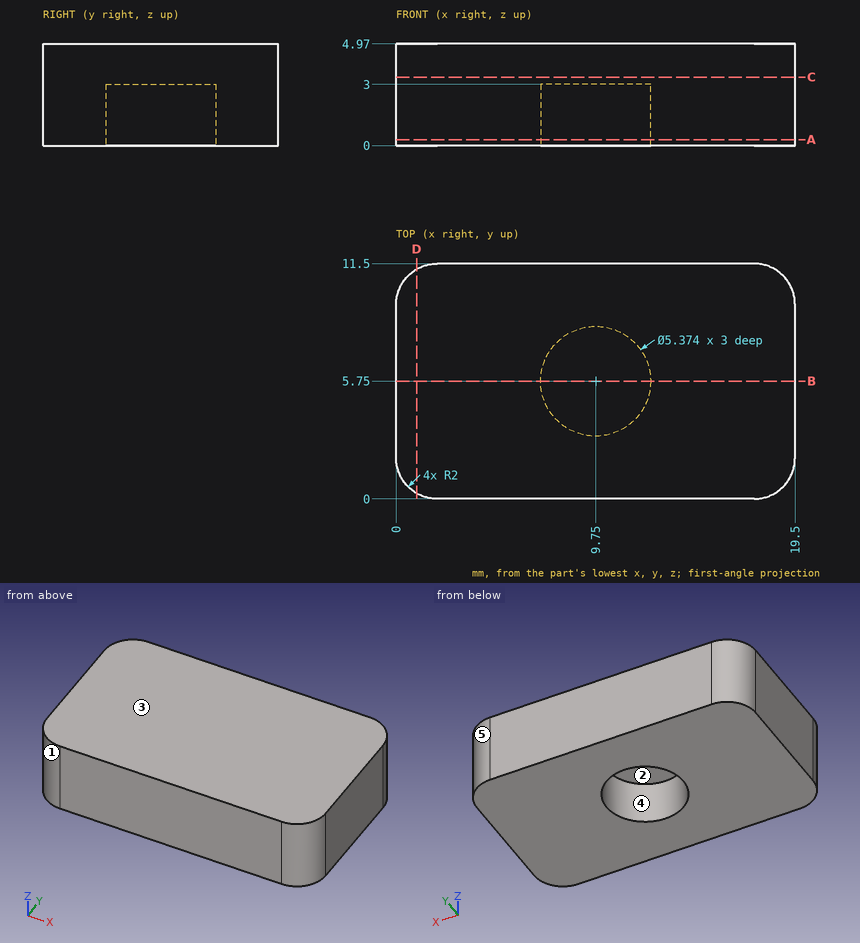
Job drawing, mm, ordinate dimensions from the low corner. One solid piece. A direction names the side the tool comes from. Coordinates: 2 decimals unless noted, no trailing zeros. Write each loop counter-clockwise with the first axis right and the second up, starting at its lowest first coordinate (ties: lowest second). Pieces come first, ordered by that corner, then holes.
Item 1: Probe line 1 (X direction, y = 5.75, z = 1.45); line 2 (Y direction, x = 9.75, z = 2.2); line 3 (Z direction, x = 8.75, y = 6). List the from-to ranges inside material, lowest first.
Item 2: Slice it at B-B (y = 5.75). Write the cut outline in (x, z).
Item 3: Pin check, flat tips, straight feed: pin 1 (6 mm diameter, centred on x = 15, y = 5, fed in from -Z); pin 2 (1.6 mm diameter, centred on x = 11, y = 6, fed in from -Z). Stop position of each tip, or through.
Item 4: Which spindle directions (+Z, -Z, +X, -X, +Y, -Y) get a long thin tool onto all of the face, cutting with end or side? Do the marked faces 1 and 2. Say none if no direction does.
Item 5: Mould opens along Y. For the marked faces 3, 4 and 5 say: released by +Y, released by -Y, zero draft, split by the parting line, or undercut.
Item 6: Slice it at A-A (z = 0.3). Write the cut outline in (x, y), and give its area (3 significant figures).
Item 7: Slice it at C-C (z = 3.35). Write the cut outline in (x, y).
Item 8: Slice it at D-D (x = 1). Write the cut outline in (y, z), and give its area (3 significant figures).
Results found:
1. line 1: x = 0 to 7.06, 12.44 to 19.5
1. line 2: y = 0 to 3.06, 8.44 to 11.5
1. line 3: z = 3 to 4.97
2. outline: (0, 0) - (7.06, 0) - (7.06, 3) - (12.44, 3) - (12.44, 0) - (19.5, 0) - (19.5, 4.97) - (0, 4.97) - close
3. pin 1: stops at z = 0
3. pin 2: stops at z = 3
4. face 1: +Z, -Z, -X, -Y
4. face 2: -Z
5. face 3: zero draft
5. face 4: undercut
5. face 5: released by +Y
6. outline: (0, 2) arc R2 ccw to (2, 0) - (17.5, 0) arc R2 ccw to (19.5, 2) - (19.5, 9.5) arc R2 ccw to (17.5, 11.5) - (2, 11.5) arc R2 ccw to (0, 9.5) - close; hole circle Ø5.37 at (9.75, 5.75)
6. area: 198 mm2
7. outline: (0, 2) arc R2 ccw to (2, 0) - (17.5, 0) arc R2 ccw to (19.5, 2) - (19.5, 9.5) arc R2 ccw to (17.5, 11.5) - (2, 11.5) arc R2 ccw to (0, 9.5) - close
8. outline: (0.27, 0) - (11.23, 0) - (11.23, 4.97) - (0.27, 4.97) - close
8. area: 54.5 mm2
